Part print with two shaded views. Sizes in mm from the minimum x, y, z corner. A direction names the side the tool comes from. Coordinates: 2 decimals unless noted, no trailing zeros. Loops run counter-clockwise (first coordinate to the right, second up) from the corner with the lowest first, then second, coordinate; pieces in that order, holes last.
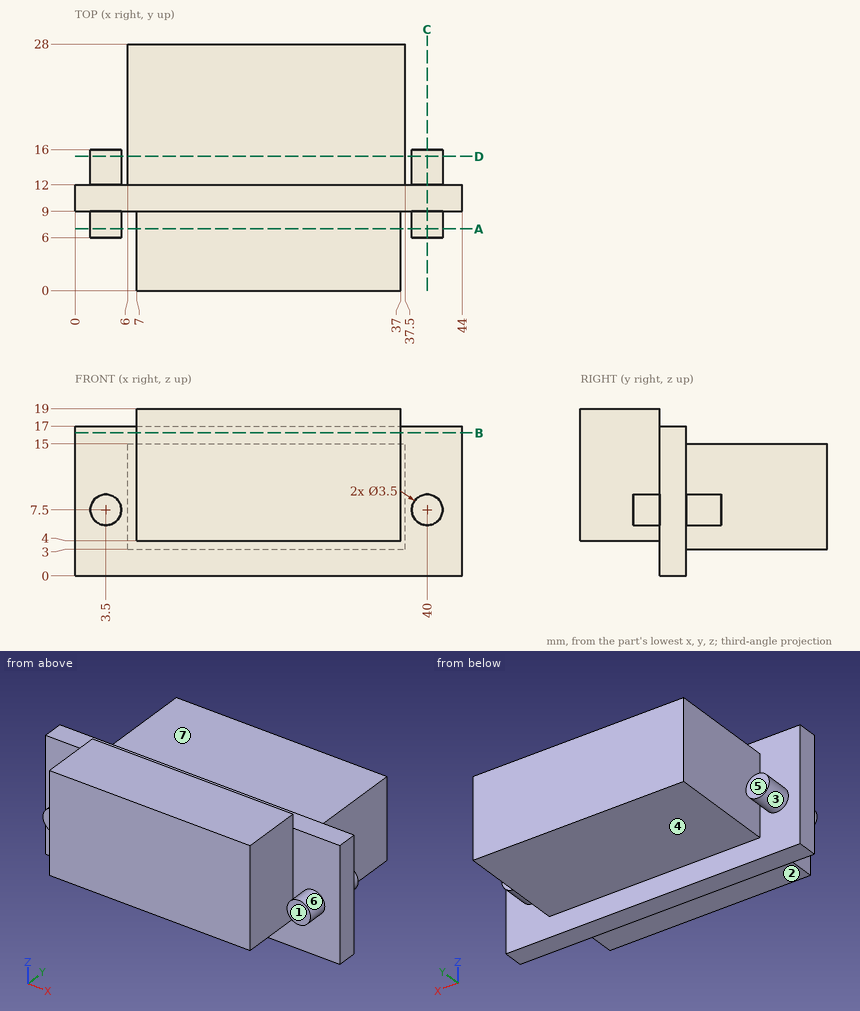
Q1. Slice it at B-B (z = 16.25). List the corners of the cut face in (x, y), and give its area (3 significant figures).
Answers:
outline: (0, 9) - (7, 9) - (7, 0) - (37, 0) - (37, 9) - (44, 9) - (44, 12) - (0, 12) - close
area: 402 mm2
Q2. Flat gauge pins, fed straight in: P1, Ø1, axis at x = 39.5, z = 7, coming from the -Y side; P2, Ø4, axis at x = 3, z = 6.5, coming from the +Y side; P3, Ø9.5, axis at y = 16, z = 10.5, coming from the +X side; P4, Ø3.5, axis at y = 19, z = 7, coming from the -X side. Where does each tip first touch, or does it go through?
Answers:
P1: stops at y = 6
P2: stops at y = 16
P3: stops at x = 44
P4: stops at x = 6
Q3. Slice it at A-A (y = 7). List the corners of the cut face in (x, z), and give its area (3 significant figures).
Answers:
outline: circle Ø3.5 at (3.5, 7.5); (7, 4) - (37, 4) - (37, 19) - (7, 19) - close; circle Ø3.5 at (40, 7.5)
area: 469 mm2
Q4. Slice it at C-C (x = 40). List the corners of the cut face in (y, z).
Answers:
outline: (6, 5.75) - (9, 5.75) - (9, 0) - (12, 0) - (12, 5.75) - (16, 5.75) - (16, 9.25) - (12, 9.25) - (12, 17) - (9, 17) - (9, 9.25) - (6, 9.25) - close
Q5. Drill centre lines: line 1 (Y direction, x = 18, z = 2.75); line 2 (Y direction, x = 13, z = 3.5); line 3 (Z direction, x = 13, y = 26.75). Where is each one in solid material? Low to high.
Answers:
line 1: y = 9 to 12
line 2: y = 9 to 28
line 3: z = 3 to 15
Q6. Mould opens along X. For the marked faces 6 and 7 say: +X half, -X half, draft (parallel to the pull), parting line (faces both ways), or undercut.
Answers:
face 6: undercut
face 7: draft
Q7. Slice it at D-D (y = 15.25). List the corners of the cut face in (x, z), and give its area (3 significant figures).
Answers:
outline: circle Ø3.5 at (3.5, 7.5); (6, 3) - (37.5, 3) - (37.5, 15) - (6, 15) - close; circle Ø3.5 at (40, 7.5)
area: 397 mm2
Q8. Which spindle directions (+Z, -Z, +X, -X, +Y, -Y) get a long thin tool onto all of the face, cutting with end or side? Do the marked faces 1, 2, 3, 4 and 5. Say none if no direction does.
Answers:
face 1: +Z, -Z, +X, -Y
face 2: -Z, +X, -X, -Y
face 3: +Y
face 4: -Z, +X, -X, +Y
face 5: +Z, -Z, -X, +Y
